from build123d import *

# Parameters (mm, degrees)
SZKIC1_R                          = 4
DODANIE_WYCI_GNI_CIE1_DEPTH       = 6
SZKIC1_3_R                        = 7
SZKIC1_3_R_2                      = 4
DODANIE_WYCI_GNI_CIE2_DEPTH       = 2
DODANIE_WYCI_GNI_CIE3_START       = 6
SZKIC1_4_R                        = 4
SZKIC1_4_R_2                      = 2.999999999999999
DODANIE_WYCI_GNI_CIE3_DEPTH       = 1
SFAZOWANIE1_SIZE                  = 0.5
SFAZOWANIE1_SIZE2                 = 0.28867513459481364
SFAZOWANIE2_SIZE                  = 0.5
SFAZOWANIE2_SIZE2                 = 0.28867513459481364
WYCI_GNI_CIE_CIENKA_CIANKA1_DEPTH = 4
WYTNIJ_WYCI_GNI_CIE1_DEPTH        = 4
WYTNIJ_WYCI_GNI_CIE2_DEPTH        = 4
ZAOKR_GLENIE2_R                   = 1
WYTNIJ_WYCI_GNI_CIE3_START        = -4
WYTNIJ_WYCI_GNI_CIE3_DEPTH        = 4
ZAOKR_GLENIE4_R                   = 0.3
ZAOKR_GLENIE5_R                   = 0.3
ZAOKR_GLENIE2_OF_LUSTRO2_R        = 1
ZAOKR_GLENIE4_OF_LUSTRO2_R        = 0.3


with BuildPart() as part:
    # Szkic1 → Dodanie-wyci_gni_cie1 (new body)
    with BuildSketch(Plane.XY):
        Circle(SZKIC1_R)
        with BuildLine():
            Line((1.5, 2.5980762113533156), (1.5, -2.5980762113533156))
            ThreePointArc((1.4999999999999998, -2.598076211353315), (-2.999999999999999, 3.7e-16), (1.4999999999999998, 2.598076211353315))
        make_face(mode=Mode.SUBTRACT)
    extrude(amount=DODANIE_WYCI_GNI_CIE1_DEPTH)

    # Szkic1_3 → Dodanie-wyci_gni_cie2 (add)
    with BuildSketch(Plane.XY):
        Circle(SZKIC1_3_R)
        Circle(SZKIC1_3_R_2, mode=Mode.SUBTRACT)
    extrude(amount=DODANIE_WYCI_GNI_CIE2_DEPTH)

    # Szkic1_4 → Dodanie-wyci_gni_cie3 (add)
    # profile 1 of 5: a face of its own
    with BuildSketch(Plane.XY.offset(DODANIE_WYCI_GNI_CIE3_START)):
        Circle(SZKIC1_4_R)
        Circle(SZKIC1_4_R_2, mode=Mode.SUBTRACT)
    # profile 2 of 5: a face of its own
    with BuildSketch(Plane.XY.offset(DODANIE_WYCI_GNI_CIE3_START)):
        with BuildLine():
            Line((1.5, 2.5980762113533156), (1.5, -2.5980762113533156))
            ThreePointArc((1.4999999999999998, -2.598076211353315), (2.5980762113533156, -1.4999999999999987), (2.999999999999999, -7.3e-16))
            ThreePointArc((2.999999999999999, 0), (2.5980762113533156, 1.4999999999999993), (1.4999999999999998, 2.598076211353315))
        make_face()
    # profile 3 of 5: a face of its own
    with BuildSketch(Plane.XY.offset(DODANIE_WYCI_GNI_CIE3_START)):
        with BuildLine():
            ThreePointArc((1.4999999999999998, 2.598076211353315), (-2.999999999999999, 3.7e-16), (1.4999999999999998, -2.598076211353315))
            Line((1.5, -2.5980762113533156), (1.5, 2.5980762113533156))
        make_face()
    # profile 4 of 5: a face of its own
    with BuildSketch(Plane.XY.offset(DODANIE_WYCI_GNI_CIE3_START)):
        with BuildLine():
            Line((1.5, 2.5980762113533156), (1.5, -2.5980762113533156))
            ThreePointArc((1.4999999999999998, -2.598076211353315), (2.5980762113533156, -1.4999999999999987), (2.999999999999999, -7.3e-16))
            ThreePointArc((2.999999999999999, 0), (2.5980762113533156, 1.4999999999999993), (1.4999999999999998, 2.598076211353315))
        make_face()
    # profile 5 of 5: a face of its own
    with BuildSketch(Plane.XY.offset(DODANIE_WYCI_GNI_CIE3_START)):
        with BuildLine():
            ThreePointArc((1.4999999999999998, 2.598076211353315), (-2.999999999999999, 3.7e-16), (1.4999999999999998, -2.598076211353315))
            Line((1.5, -2.5980762113533156), (1.5, 2.5980762113533156))
        make_face()
    extrude(amount=DODANIE_WYCI_GNI_CIE3_DEPTH)

    # Sfazowanie1
    sfazowanie1_edges = [part.edges().sort_by_distance(p)[0] for p in [
        (1.5, 0, 6),
        (-2.999999999999999, 8.9e-16, 6),
    ]]
    sfazowanie1_side = [part.faces().sort_by_distance(p)[0] for p in [
        (-0.5139804124502736, 6.2e-16, 6),
    ]]
    chamfer(sfazowanie1_edges, length=SFAZOWANIE1_SIZE, length2=SFAZOWANIE1_SIZE2, reference=sfazowanie1_side[0])

    # Sfazowanie2
    sfazowanie2_edges = [part.edges().sort_by_distance(p)[0] for p in [
        (-4, 4.9e-16, 7),
    ]]
    sfazowanie2_side = [part.faces().sort_by_distance(p)[0] for p in [
        (-4, 4.9e-16, 4.5),
    ]]
    chamfer(sfazowanie2_edges, length=SFAZOWANIE2_SIZE, length2=SFAZOWANIE2_SIZE2, reference=sfazowanie2_side[0])

    # Szkic3 → Wyci_gni_cie-cienka _cianka1 (add)
    with BuildSketch(Plane.XY.offset(2)):
        Polygon((0.9907558800275146, -3.8680137479259677), (1.811604224009121, -6.123276037812147), (2.751296844795029, -5.781255894486478), (1.930448500813423, -3.5259936046002984), align=None)
        Polygon((-1.930448500813423, -3.525993604600299), (-2.7512968447950286, -5.7812558944864785), (-1.81160422400912, -6.123276037812148), (-0.9907558800275145, -3.868013747925968), align=None)
    wyci_gni_cie_cienka_cianka1 = extrude(amount=WYCI_GNI_CIE_CIENKA_CIANKA1_DEPTH)

    # Szkic4 → Wytnij-wyci_gni_cie1 (cut)
    with BuildSketch(Plane(origin=(-0.5713964233589274, 0.2079712900688191, 0), x_dir=(0, 0, 1), z_dir=(-0.9396926207859082, 0.3420201433256693, 0))):
        Polygon((6, -6.373602444112237), (6, -5.623602444112237), (2, -6.373602444112238), align=None)
    wytnij_wyci_gni_cie1 = extrude(amount=-WYTNIJ_WYCI_GNI_CIE1_DEPTH, mode=Mode.SUBTRACT)

    # Szkic5 → Wytnij-wyci_gni_cie2 (cut)
    with BuildSketch(Plane(origin=(-0.36829619742698255, -0.13404885325685056, 0), x_dir=(0, 0, 1), z_dir=(-0.939692620785908, -0.3420201433256696, 0))):
        Polygon((2, -6.373602444112238), (6, -6.373602444112237), (6, -5.373602444112237), align=None)
    wytnij_wyci_gni_cie2 = extrude(amount=-WYTNIJ_WYCI_GNI_CIE2_DEPTH, mode=Mode.SUBTRACT)

    # Zaokr_glenie2
    zaokr_glenie2_edges = [part.edges().sort_by_distance(p)[0] for p in [
        (-2.0249354269078235, -5.247496500559882, 6),
        (1.9394303910764068, -5.012573345363405, 6),
    ]]
    fillet(zaokr_glenie2_edges, radius=ZAOKR_GLENIE2_R)

    # Szkic6 → Wytnij-wyci_gni_cie3 (cut)
    with BuildSketch(Plane.XY.offset(2).offset(WYTNIJ_WYCI_GNI_CIE3_START)):
        with BuildLine():
            Line((-1.8116042240091212, -6.12327603781215), (-2.0220891373099885, -6.701578584242144))
            ThreePointArc((-2.0220891373099885, -6.701578584242144), (-0.0188863375955117, -6.999974521828791), (1.985897465033318, -6.7123923647515005))
            Line((1.985897465033318, -6.7123923647515005), (1.8116042240091235, -6.12327603781215))
            Line((1.8116042240091235, -6.12327603781215), (0.9932012722690525, -3.8747324078913032))
            ThreePointArc((0.9932012722690525, -3.8747324078913032), (-9e-16, -3.999999999999983), (-0.9932012722690527, -3.874732407891303))
            Line((-0.9932012722690527, -3.874732407891303), (-1.8116042240091212, -6.12327603781215))
        make_face()
    extrude(amount=WYTNIJ_WYCI_GNI_CIE3_DEPTH, mode=Mode.SUBTRACT)

    # Zaokr_glenie4
    zaokr_glenie4_edges = [part.edges().sort_by_distance(p)[0] for p in [
        (2.281450534402075, -5.952265966149312, 2),
        (-2.281450534402074, -5.952265966149313, 2),
    ]]
    fillet(zaokr_glenie4_edges, radius=ZAOKR_GLENIE4_R)

    # Zaokr_glenie5
    zaokr_glenie5_edges = [part.edges().sort_by_distance(p)[0] for p in [
        (0.0188863375955115, 6.999974521828793, 2),
    ]]
    fillet(zaokr_glenie5_edges, radius=ZAOKR_GLENIE5_R)

    # Lustro2: Wyci_gni_cie-cienka _cianka1, Wytnij-wyci_gni_cie1, Wytnij-wyci_gni_cie2 across plane
    add(wyci_gni_cie_cienka_cianka1.mirror(Plane.ZX))
    add(wytnij_wyci_gni_cie1.mirror(Plane.ZX), mode=Mode.SUBTRACT)
    add(wytnij_wyci_gni_cie2.mirror(Plane.ZX), mode=Mode.SUBTRACT)

    # Zaokr_glenie2 of Lustro2
    zaokr_glenie2_of_lustro2_edges = [part.edges().sort_by_distance(p)[0] for p in [
        (-2.0249354269078235, 5.247496500559882, 6),
        (1.9394303910764068, 5.012573345363405, 6),
    ]]
    fillet(zaokr_glenie2_of_lustro2_edges, radius=ZAOKR_GLENIE2_OF_LUSTRO2_R)

    # Zaokr_glenie4 of Lustro2
    zaokr_glenie4_of_lustro2_edges = [part.edges().sort_by_distance(p)[0] for p in [
        (2.281450534402075, 5.952265966149312, 2),
        (-2.281450534402074, 5.952265966149313, 2),
    ]]
    fillet(zaokr_glenie4_of_lustro2_edges, radius=ZAOKR_GLENIE4_OF_LUSTRO2_R)


solid = part.part
Read the model definition and answer for the solid it produces. Units are mm, in the model's axes. A direction names the side the tool comes from. Round coordinates to 2 decimals unless told otherwise and drop trailing zeros. Write each loop counter-clockwise with the first axis right and the second up, starting at its lowest first coordinate (ties: lowest second). Pieces come first, ordered by that corner, then holes.
1. Determine the mould class of faces 4 (the face through (-1.35, 4.86, 3.97)), 5 (the face through (-2.276, -4.477, 3.972)), 6 (the face through (2.29, 4.51, 3.97)) for opening direction X: pulls with the +X half, pulls with the -X half, needs draft (parallel to the pull), parting line crosses it, or undercut.
2. The part is cut by section C-C, the plane y = 0. Determine the outline of the cut face in (x, z), then the cut area to 3 significant figures.
3. The part is cut by section D-D, the plane z = 2.5. Determine the outline of the cut face in (x, y).
4. Given pin 1 Ø4 at (y, z) = (-3, 1.5) entering from +X; pin 2 Ø0.9 at (x, y) = (-1.5, -4) entering from +Z; pin 3 Ø2 at (y, z) = (4, 6) entering from -X, each flat-ended and moving along its own axis, determine where each tip first touches the part or whether it passes through.
5. The part is cut by section A-A, the plane z = 0.5. Determine the outline of the cut face in (x, y), then the cut area to 3 significant figures.
6. The part is cut by section B-B, the plane x = 0. Determine the outline of the cut face in (y, z).
7. Straight lines are drawn through the part: L1, parallel to Y at x = 0, z = 1.25; L2, parallel to Y at x = 0, z = 3.5; L3, parallel to Z at x = -4.75, y = -4. For each, find the intervals that lie inside material, in ascending order.
8. Which of the six approach directions +Z, -Z, +X, -X, +Y, -Y give full straight-line access (tool end or side, diameter ignored) to faces 1 (the face through (1.6, 4, 6)), 2 (the face through (1.5, 0, 3)), 3 (the face through (-1.6, -4.1, 6))?
Values:
1. face 4: undercut
1. face 5: pulls with the -X half
1. face 6: pulls with the +X half
2. outline: (-7, 0) - (-3, 0) - (-3, 5.71) - (-2.5, 6) - (1, 6) - (1.5, 5.71) - (1.5, 0) - (7, 0) - (7, 1.7) arc R0.3 ccw to (6.7, 2) - (4, 2) - (4, 6.5) - (3.71, 7) - (-3.71, 7) - (-4, 6.5) - (-4, 2) - (-6.7, 2) arc R0.3 ccw to (-7, 1.7) - close
2. area: 41.0 mm2
3. outline: (-2.72, -5.69) - (-1.78, -6.04) - (-0.99, -3.87) arc R4 ccw to (0.99, -3.87) - (1.77, -6.01) - (2.71, -5.66) - (1.93, -3.53) - (1.79, -3.58) arc R4 ccw to (1.79, 3.58) - (1.93, 3.53) - (2.71, 5.66) - (1.77, 6.01) - (0.99, 3.87) arc R4 ccw to (-0.99, 3.87) - (-1.78, 6.04) - (-2.72, 5.69) - (-1.93, 3.53) - (-1.79, 3.58) arc R4 ccw to (-1.79, -3.58) - (-1.93, -3.53) - close; hole (1.5, -2.6) - (1.5, 2.6) arc R3 ccw (long way) to start
4. pin 1: stops at x = 6.93
4. pin 2: stops at z = 6.81
4. pin 3: stops at x = -2.65
5. outline: (-2.02, -6.7) - (-0.99, -3.87) arc R4 ccw to (0.99, -3.87) - (1.81, -6.12) - (1.99, -6.71) arc R7 ccw (long way) to start; hole (1.5, -2.6) - (1.5, 2.6) arc R3 ccw (long way) to start
5. area: 122 mm2
6. outline: (-4, 0) - (-3, 0) - (-3, 5.71) - (-2.5, 6) - (2.5, 6) - (3, 5.71) - (3, 0) - (7, 0) - (7, 1.7) arc R0.3 ccw to (6.7, 2) - (4, 2) - (4, 6.5) - (3.71, 7) - (-3.71, 7) - (-4, 6.5) - close
7. L1: y = -4 to -3, 3 to 7
7. L2: y = -4 to -3, 3 to 4
7. L3: z = 0 to 2
8. face 1: +Z, +X, +Y
8. face 2: -Z
8. face 3: +Z, -X, -Y
